Input: part model. Units: mm. Frame: model coordinates. Face numbers are marked on the shaded views. A direction names the side the tool comes from. Give positions to 0.01 mm unless a question says otherwise; leave off trailing zeros. Loops run counter-clockwise (first coordinate to the right, second up) from the corner with the lowest first, then second, coordinate; pieces in that order, holes last. Notation, with made-up numbers: (51, -26.5) -> (82, -26.5) arc R18 cw to (82, 1.5) -> close; hole circle Ø10 at (58.5, 86.5). An arc over 180 degrees is marked (long way). Answer as a JSON object with one key per item and string values.
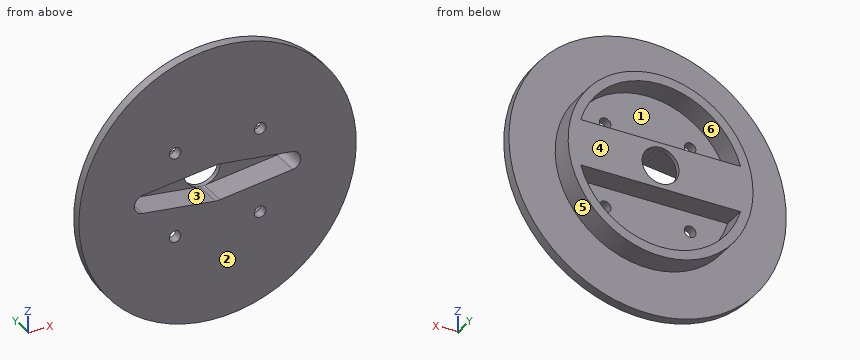
```python
from build123d import *

# Parameters (mm, degrees)
SKETCH_1_R          = 30
SKETCH_1_R_2        = 1.25
EXTRUDE_1_DEPTH     = 2
SKETCH_2_R          = 20
EXTRUDE_2_DEPTH     = 5
CUT_EXTRUDE_1_DEPTH = 6
SKETCH_5_R          = 4
CUT_EXTRUDE_2_DEPTH = 6


with BuildPart() as part:
    # 草图1 → 凸台-拉伸1 (new body)
    with BuildSketch(Plane(origin=(0, 0, 0), x_dir=(1, 0, 0), z_dir=(0, 1, 0))):
        with Locations(Location((0, 0, 0), (0, 0, 270))):
            Circle(SKETCH_1_R)
        with Locations(Location((9.192388155, 9.192388155, 0), (0, 0, 270))):
            Circle(SKETCH_1_R_2, mode=Mode.SUBTRACT)
        with Locations(Location((9.192388155, -9.192388155, 0), (0, 0, 270))):
            Circle(SKETCH_1_R_2, mode=Mode.SUBTRACT)
        with Locations(Location((-9.192388155, -9.192388155, 0), (0, 0, 270))):
            Circle(SKETCH_1_R_2, mode=Mode.SUBTRACT)
        with Locations(Location((-9.192388155, 9.192388155, 0), (0, 0, 270))):
            Circle(SKETCH_1_R_2, mode=Mode.SUBTRACT)
    extrude(amount=EXTRUDE_1_DEPTH)

    # 草图2 → 凸台-拉伸2 (add)
    with BuildSketch(Plane(origin=(0, 2, 0), x_dir=(1, 0, 0), z_dir=(0, 1, 0))):
        with Locations(Location((0, 0, 0), (0, 0, 270))):
            Circle(SKETCH_2_R)
        with BuildLine():
            Line((-17.291616466, 5), (17.291616466, 5))
            ThreePointArc((17.291616466, 5), (0, 18), (-17.291616466, 5))
        make_face(mode=Mode.SUBTRACT)
        with BuildLine():
            Line((-17.291616466, -5), (17.291616466, -5))
            ThreePointArc((17.291616466, -5), (0, -18), (-17.291616466, -5))
        make_face(mode=Mode.SUBTRACT)
    extrude(amount=EXTRUDE_2_DEPTH)

    # 草图4 → 切除-拉伸1 (cut)
    with BuildSketch(Plane(origin=(0, 0, 0), x_dir=(-1, 0, 0), z_dir=(0, -1, 0))):
        with BuildLine():
            Line((-0.5, -3.968626967), (-16.25, -1.984313483))
            ThreePointArc((-16.25, -1.984313483), (-18, 0), (-16.25, 1.984313483))
            Line((-16.25, 1.984313483), (-0.5, 3.968626967))
            ThreePointArc((-0.5, 3.968626967), (0, 4), (0.5, 3.968626967))
            Line((0.5, 3.968626967), (16.25, 1.984313483))
            ThreePointArc((16.25, 1.984313483), (18, 0), (16.25, -1.984313483))
            Line((16.25, -1.984313483), (0.5, -3.968626967))
            ThreePointArc((0.5, -3.968626967), (0, -4), (-0.5, -3.968626967))
        make_face()
    extrude(amount=-CUT_EXTRUDE_1_DEPTH, mode=Mode.SUBTRACT)

    # 草图5 → 切除-拉伸2 (cut)
    with BuildSketch(Plane(origin=(0, 6, 0), x_dir=(-1, 0, 0), z_dir=(0, -1, 0))):
        with Locations(Location((0, 0, 0), (0, 0, 97.180755781))):
            Circle(SKETCH_5_R)
    extrude(amount=-CUT_EXTRUDE_2_DEPTH, mode=Mode.SUBTRACT)


solid = part.part
```
Q1. Section A-A, the plane z = 0. Return the cut outline in (x, y).
Evaluation:
{"outline": "(-30, 0) -> (-18, 0) -> (-18, 6) -> (-4, 6) -> (-4, 7) -> (-20, 7) -> (-20, 2) -> (-30, 2) -> close; (4, 6) -> (18, 6) -> (18, 0) -> (30, 0) -> (30, 2) -> (20, 2) -> (20, 7) -> (4, 7) -> close"}
Q2. Section D-D, the plane z = 23.5. Return the cut outline in (x, y).
Evaluation:
{"outline": "(-18.65, 0) -> (18.65, 0) -> (18.65, 2) -> (-18.65, 2) -> close"}
Q3. Section B-B, the plane y = 3. Return the cut outline in (x, z), then the cut area to 3 significant figures.
Evaluation:
{"outline": "circle Ø40 at (0, 0); hole (-17.29, -5) arc R18 ccw to (17.29, -5) -> close; hole (-17.29, 5) -> (17.29, 5) arc R18 ccw to start; hole (-16.25, -1.98) -> (-0.5, -3.97) arc R4 ccw to (0.5, -3.97) -> (16.25, -1.98) arc R2 ccw to (16.25, 1.98) -> (0.5, 3.97) arc R4 ccw to (-0.5, 3.97) -> (-16.25, 1.98) arc R2 ccw to start", "area": "388 mm2"}
Q4. Draft query along X for the marked faces 4, 5 and 6. Return one class per face: +X half, -X half, draft (parallel to the pull), parting line (faces both ways), or undercut.
Evaluation:
{"face 4": "draft", "face 5": "parting line", "face 6": "undercut"}
Q5. Pin query (flat end, axial travel): pin 1 (6.5 mm diameter, centred on x = 0, z = 0, fed in from +Y); pin 2 (3 mm diameter, centred on x = 9.19, z = 9.19, fed in from +Y); pin 3 (2 mm diameter, centred on x = 9, y = 4.5, fed in from -Z); pin 4 (2.5 mm diameter, centred on x = -12, z = 1, fed in from -Y). Return the tip coordinate at first contact, or that it passes through.
Evaluation:
{"pin 1": "passes through", "pin 2": "stops at y = 2", "pin 3": "stops at z = -18.33", "pin 4": "stops at y = 6"}
Q6. Access query for the marked faces 1, 2 and 3. Directions: +Z, -Z, +X, -X, +Y, -Y. A direction counts if a zero-diameter tool reaches every point of the face in a straight line with its end or side. Return the directions, or none.
Evaluation:
{"face 1": "+Y", "face 2": "+Z, -Z, +X, -X, -Y", "face 3": "-Y"}
Q7. Section C-C, the plane x = -7. Return the cut outline in (y, z) (3 decimals).
Evaluation:
{"outline": "(0, -29.172) -> (2, -29.172) -> (2, -18.735) -> (7, -18.735) -> (7, -16.583) -> (2, -16.583) -> (2, -5) -> (7, -5) -> (7, 5) -> (2, 5) -> (2, 16.583) -> (7, 16.583) -> (7, 18.735) -> (2, 18.735) -> (2, 29.172) -> (0, 29.172) -> (0, 3.15) -> (6, 3.15) -> (6, -3.15) -> (0, -3.15) -> close"}
Q8. Ray query, line 1 along Z through (x, y) = (-15, 5); line 2 along Z through (x, y) = (16.5, 6.5); line 3 along Z through (x, y) = (-6, 5.5). Return the intervals inside material, ascending.
Evaluation:
{"line 1": "z = -13.23 to -9.95, -5 to -2.14, 2.14 to 5, 9.95 to 13.23", "line 2": "z = -11.3 to -7.19, -5 to 5, 7.19 to 11.3", "line 3": "z = -19.08 to -16.97, -5 to -3.28, 3.28 to 5, 16.97 to 19.08"}
